The listing builds one solid part. Answer for the finished solid, in the listing's coordinates (mm). Face numbers are marked on the shaded views. A direction names the side the tool comes from. Give positions to 0.01 mm unless a question says otherwise; leave off trailing zeros. Loops run counter-clockwise (first coordinate to the right, second up) from the corner with the lowest first, then second, coordinate; pieces in that order, holes last. Notation, with made-up numbers: M 77.5,31 L 105.5,31 A29 cw 105.5,63 Z; hole C 83,25.25 d2. An arc over 180 degrees is marked long. Return JSON: item names as keys, results as strings.
from build123d import *

# Parameters (mm, degrees)
SKETCH7_W               = 45
SKETCH7_H               = 45
SKETCH7_R               = 1.875
SKETCH7_R_2             = 14
SKETCH7_R_3             = 4.5
BOSS_EXTRUDE5_DEPTH     = 5
SKETCH7_3_W             = 45
SKETCH7_3_H             = 2
BOSS_EXTRUDE6_DEPTH     = 40
BOSS_EXTRUDE7_DEPTH     = 5
SKETCH7_4_W             = 45
SKETCH7_4_H             = 8
BOSS_EXTRUDE8_DEPTH     = 40
SKETCH10_R              = 2.375
CUT_EXTRUDE2_DEPTH      = 9
CUT_EXTRUDE2_DEPTH_BACK = 5


with BuildPart() as part:
    # Sketch7 → Boss-Extrude5 (new body)
    with BuildSketch(Plane(origin=(0, 0, 0), x_dir=(1, 0, 0), z_dir=(0, 1, 0))):
        with Locations((5.756289545, -118.050969126)):
            Rectangle(SKETCH7_W, SKETCH7_H)
        with Locations((5.756289545, -136.050969126)):
            Circle(SKETCH7_R, mode=Mode.SUBTRACT)
        with Locations((5.362034713, -118.985312035)):
            Circle(SKETCH7_R_2, mode=Mode.SUBTRACT)
        with Locations((5.756289545, -101.050969126)):
            Circle(SKETCH7_R, mode=Mode.SUBTRACT)
        with Locations((5.362034713, -118.985312035)):
            Circle(SKETCH7_R_2)
        with Locations((12.756289545, -118.550969126)):
            Circle(SKETCH7_R_3, mode=Mode.SUBTRACT)
    extrude(amount=BOSS_EXTRUDE5_DEPTH)

    # Sketch7<3> → Boss-Extrude6 (add)
    with BuildSketch(Plane(origin=(0, 0, 0), x_dir=(1, 0, 0), z_dir=(0, 1, 0))):
        with Locations((5.756289545, -141.550969126)):
            Rectangle(SKETCH7_3_W, SKETCH7_3_H)
    extrude(amount=BOSS_EXTRUDE6_DEPTH)

    # Sketch8 → Boss-Extrude7 (add)
    with BuildSketch(Plane.ZY.offset(16.743710455)):
        Polygon((140.550969126, 11), (140.550969126, 5), (121.550969126, 5), (140.550969126, 19), align=None)
    boss_extrude7 = extrude(amount=-BOSS_EXTRUDE7_DEPTH)

    # Mirror2: Boss-Extrude7 across plane
    add(boss_extrude7.mirror(Plane.ZY.offset(-5.756289545)))

    # Sketch7<4> → Boss-Extrude8 (add)
    with BuildSketch(Plane(origin=(0, 0, 0), x_dir=(1, 0, 0), z_dir=(0, 1, 0))):
        with Locations((5.756289545, -146.550969126)):
            Rectangle(SKETCH7_4_W, SKETCH7_4_H)
    extrude(amount=BOSS_EXTRUDE8_DEPTH)

    # Sketch10 → Cut-Extrude2 (cut, two sides)
    with BuildSketch(Plane.XY.offset(142.550969126)) as cut_extrude2_sk:
        with Locations((21.756289545, 27)):
            Circle(SKETCH10_R)
        with Locations((-10.243710455, 27)):
            Circle(SKETCH10_R)
    extrude(amount=CUT_EXTRUDE2_DEPTH, mode=Mode.SUBTRACT)
    extrude(cut_extrude2_sk.sketch, amount=-CUT_EXTRUDE2_DEPTH_BACK, mode=Mode.SUBTRACT)


solid = part.part
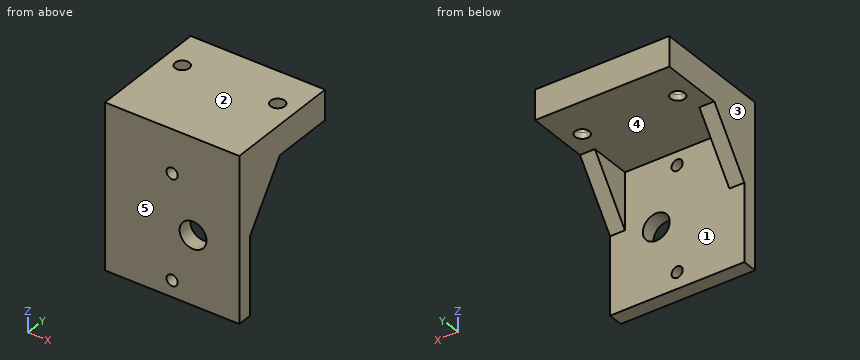
(1) The part is cut by section A-A (y = 27). Determine the outline of the cut face in (x, z), and give its area (3 significant figures).
Values follow:
{"outline": "M -16.74,140.55 L -12.62,140.55 L -12.62,150.55 L -16.74,150.55 Z; M -7.87,140.55 L 19.38,140.55 L 19.38,150.55 L -7.87,150.55 Z; M 24.13,140.55 L 28.26,140.55 L 28.26,150.55 L 24.13,150.55 Z", "area": "355 mm²"}
(2) The part is cut by section B-B (x = 20.5). Determine the outline of the cut face in (y, z), and give its area (3 significant figures).
Values follow:
{"outline": "M 0,95.55 L 5,95.55 L 5,140.55 L 24.98,140.55 L 24.98,150.55 L 0,150.55 Z; M 29.02,140.55 L 40,140.55 L 40,150.55 L 29.02,150.55 Z", "area": "585 mm²"}
(3) The part is cut by section C-C (z = 130.5). Determine the outline of the cut face in (x, y).
Values follow:
{"outline": "M -16.74,0 L 28.26,0 L 28.26,11.59 L 23.26,11.59 L 23.26,5 L -11.74,5 L -11.74,11.59 L -16.74,11.59 Z"}
(4) Determine the mould class of the marked faces 1, 2 and 3 for opening direction X: released by +X, released by -X, zero draft, split by the parting line, or undercut.
Values follow:
{"face 1": "undercut", "face 2": "zero draft", "face 3": "released by -X"}
(5) A tool of negligible diameter and unlimited length cuts with its end or side. For the marked faces 4 and 5, from which of +Z, -Z, +X, -X, +Y, -Y can it reach the whole face along a straight path? Write none if from no direction.
Values follow:
{"face 4": "-Z, +Y", "face 5": "+Z, -Z, +X, -X, -Y"}
(6) Given pin 1 (10.5 mm diameter, centred on x = 8, y = 19, fed in from -Z); pin 2 (7 mm diameter, centred on y = 15, z = 127.5, fed in from +X); pin 3 (8 mm diameter, centred on x = 18, z = 108, fed in from +Y), each flat-ended and moving along its own axis, determine where each tip first touches the part or whether it passes through.
Values follow:
{"pin 1": "z = 140.55", "pin 2": "through", "pin 3": "y = 5"}
(7) Straight lines are drawn through the part: line 1 along X through (y, z) = (27, 147.75); line 2 along X through (y, z) = (28.5, 143.5); line 3 along Z through (x, y) = (9, 8.5). For each, find the intervals that lie inside material, in ascending order.
Values follow:
{"line 1": "-16.74 to -12.62, -7.87 to 19.38, 24.13 to 28.26", "line 2": "-16.74 to -12.09, -8.4 to 19.91, 23.6 to 28.26", "line 3": "140.55 to 150.55"}
(8) The part is cut by section D-D (y = 18). Determine the outline of the cut face in (x, z), and give its area (3 significant figures).
Values follow:
{"outline": "M -16.74,139.19 L -11.74,139.19 L -11.74,140.55 L 23.26,140.55 L 23.26,139.19 L 28.26,139.19 L 28.26,150.55 L -16.74,150.55 Z", "area": "464 mm²"}
